Could you check a few things on this model? Use its own coordinates, in mm. Face numbers are marked on the shaded views. A direction names the side the tool comes from. Round coordinates to 2 decimals unless told otherwise and drop trailing zeros. Loops run counter-clockwise (first coordinate to the right, second up) from the corner with the lowest first, then second, coordinate; pieces in that order, holes last. Notation, with made-up numbers: M 2.25,24.5 L 12.25,24.5 A26 cw 12.25,52.5 Z; hole C 76,-21 d10. An arc over 180 degrees is marked long. One line per item, written item: value. Start each with the question number.
Q1. Imagine slicing it at A-A (z = 1.1). Please give me the cut outline in (x, y).
Q2. Please list where these lines run through material, in increasing order: line 1 along X through (y, z) = (3.5, 0.85); line 2 along X through (y, z) = (6.5, 4.1); line 3 along X through (y, z) = (12.5, 2.6).
Q3. I'm going to push flat-ended pins straight in: pin 1 Ø1 at (x, z) = (-4.5, 4.5) entering from +Y; pin 2 Ø1 at (x, z) = (-6.5, 4) entering from +Y; pin 3 Ø8 at (x, y) = (5, 3.5) entering from +Z. Where does each tip first touch, or does it pass through?
Q4. Which directions (+Z, -Z, +X, -X, +Y, -Y) give clear straight access to the entire face, cutting with the end or side of a thin tool? Please do the marked faces 1 and 2.
Q5. Imagine slicing it at B-B (y = 15.5). Please give me the cut outline in (x, z).
Q6. Imagine slicing it at D-D (y = -1.5). Please give me the cut outline in (x, z).
Q7. Thinking about a two-plate mould opening in X: for the marked faces 3, 4 and 5, which applies, released by +X, released by -X, zero draft, split by the parting line, or undercut?
Q8. Imagine slicing it at C-C (x = 3). Please give me the cut outline in (y, z).
from build123d import *

# Parameters (mm, degrees)
F1_DEPTH    = 5.1
F2_T1_DEPTH = 7.5361277396
F2_T3_DEPTH = 7.6009429286


# Not quite as in the source:
# - a fillet or chamfer that OpenCascade refuses, or shapes differently, is made with other operations: its cross-section is extruded or revolved along the edge and cut away or added


with BuildPart() as f1:
    # F0 (on Top) → F1 (new body)
    with BuildSketch(Plane.XY):
        with BuildLine():
            Line((0.0307608464, 20.8328839523), (-9.3844581437, 5.9280642161))
            ThreePointArc((-9.3844581437, 5.9280642161), (-3.6624820561, 10.4783693955), (3.6482130412, 10.4833459165))
            ThreePointArc((3.6482130412, 10.4833459165), (-0.6590930389, 14.7847915444), (0.0307608464, 20.8328839523))
        make_face()
        with BuildLine():
            ThreePointArc((-8.0650120901, -0.752050521), (-0.3764319792, 8.0912482946), (8.1, 0))
            ThreePointArc((8.1, 0), (6.8438750945, -4.3325943371), (3.465092916, -7.3214159207))
            Line((3.465092916, -7.3214159207), (4.7484606627, -10.0330514468))
            ThreePointArc((4.7484606627, -10.0330514468), (9.0496936401, -6.4275224637), (11.0372396512, -1.1787030508))
            ThreePointArc((11.0372396512, -1.1787030508), (11.084298808, -0.5901863569), (11.1, 0))
            ThreePointArc((11.1, 0), (9.0472417, 6.4309733028), (3.6482130412, 10.4833459165))
            ThreePointArc((3.6482130412, 10.4833459165), (-3.6624820561, 10.4783693955), (-9.3844581437, 5.9280642161))
            ThreePointArc((-9.3844581437, 5.9280642161), (-10.7943717933, 2.586800647), (-11.052053605, -1.030587751))
            Line((-11.052053605, -1.030587751), (-8.0650120901, -0.752050521))
        make_face()
        with BuildLine():
            ThreePointArc((11.1, 0), (11.084298808, -0.5901863569), (11.0372396512, -1.1787030508))
            Line((11.0372396512, -1.1787030508), (12.9093090053, 16.351138829))
            ThreePointArc((12.9093090053, 16.351138829), (9.6953604205, 11.1814335847), (3.6482130412, 10.4833459165))
            ThreePointArc((3.6482130412, 10.4833459165), (9.0472417, 6.4309733028), (11.1, 0))
        make_face()
        with BuildLine():
            ThreePointArc((0.0307608464, 20.8328839523), (-0.6590930389, 14.7847915444), (3.6482130412, 10.4833459165))
            ThreePointArc((3.6482130412, 10.4833459165), (9.6953604205, 11.1814335847), (12.9093090053, 16.351138829))
            ThreePointArc((12.9093090053, 16.351138829), (12.938985951, 16.7222754829), (12.9488876036, 17.0944650773))
            ThreePointArc((12.9488876036, 17.0944650773), (12.7292523894, 18.8341930364), (12.0841294975, 20.4647479889))
            Line((12.0841294975, 20.4647479889), (9.4547401144, 19.0203410268))
            ThreePointArc((9.4547401144, 19.0203410268), (9.8233817669, 18.0885953396), (9.9488876036, 17.0944650773))
            ThreePointArc((9.9488876036, 17.0944650773), (4.5409128854, 13.3504555697), (2.9400840071, 19.730200443))
            Line((2.9400840071, 19.730200443), (0.6834813098, 21.7070019672))
            ThreePointArc((0.6834813098, 21.7070019672), (0.3400665642, 21.282677888), (0.0307608464, 20.8328839523))
        make_face()
    extrude(amount=F1_DEPTH)

    # F2: chamfer of 0.5 on 4 edges, made by hand

    # F2_s2 → F2_t1 (cut)
    with BuildSketch(Plane.XY.offset(-1.2180638698)):
        with BuildLine():
            Line((9.8685498702, 19.2476598469), (9.6470180572, 18.6188768158))
            ThreePointArc((9.6470180572, 18.6188768158), (9.5595268283, 18.8158843724), (9.4547401144, 19.0203410268))
            Line((9.4547401144, 19.0203410268), (9.8685498702, 19.2476598469))
        make_face()
        with BuildLine():
            Line((2.665855064, 19.3795684325), (2.5849429173, 20.0413068015))
            Line((2.5849429173, 20.0413068015), (2.9400840071, 19.730200443))
            ThreePointArc((2.9400840071, 19.730200443), (2.7937225781, 19.5531097571), (2.665855064, 19.3795684325))
        make_face()
    extrude(amount=F2_T1_DEPTH, mode=Mode.SUBTRACT)

    # F2_s4 → F2_t3 (cut)
    with BuildSketch(Plane.XY.offset(-1.2504714643)):
        with BuildLine():
            Line((3.8848953119, -7.1075726106), (3.6727644101, -7.7602062851))
            Line((3.6727644101, -7.7602062851), (3.465092916, -7.3214159207))
            ThreePointArc((3.465092916, -7.3214159207), (3.682856675, -7.2143306489), (3.8848953119, -7.1075726106))
        make_face()
        with BuildLine():
            Line((-8.5483679919, -0.7971227482), (-8.0950937203, -0.2818823506))
            ThreePointArc((-8.0950937203, -0.2818823506), (-8.0839209794, -0.5101192), (-8.0650120901, -0.752050521))
            Line((-8.0650120901, -0.752050521), (-8.5483679919, -0.7971227482))
        make_face()
    extrude(amount=F2_T3_DEPTH, mode=Mode.SUBTRACT)


solid = f1.part
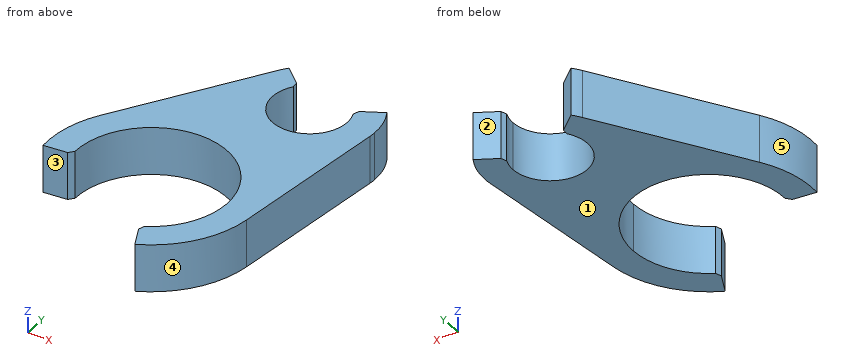
Report:
1. outline: M -11.05,-1.03 L -8.55,-0.8 L -8.1,-0.28 A8.1 cw long 3.88,-7.11 L 3.67,-7.76 L 4.75,-10.03 A11.1 ccw 11.04,-1.18 L 12.91,16.35 A7 ccw 12.08,20.46 L 9.87,19.25 L 9.65,18.62 A4 cw long 2.67,19.38 L 2.58,20.04 L 0.68,21.71 A7 ccw 0.03,20.83 L -9.38,5.93 A11.1 ccw Z
2. line 1: x = -10.53 to -7.3, 7.3 to 11.54
2. line 2: x = -9.02 to -4.83, 4.83 to 11.86
2. line 3: x = -5.23 to 12.5
3. pin 1: stops at y = 14.45
3. pin 2: stops at y = 11.29
3. pin 3: stops at z = 5.1
4. face 1: -Z, +X, -X, +Y, -Y
4. face 2: +Z, -Z, +Y
5. outline: M -3.34,0 L 2.28,0 L 2.28,5.1 L -3.34,5.1 Z; M 9.62,0 L 12.82,0 L 12.82,5.1 L 9.62,5.1 Z
6. outline: M 7.96,0 L 11,0 L 11,5.1 L 7.96,5.1 Z
7. face 3: undercut
7. face 4: released by +X
7. face 5: released by -X
8. outline: M 7.52,0 L 14.39,0 L 14.39,5.1 L 7.52,5.1 Z
